Autodesk Inventor part; units mm, degrees
ref_plane "Work Plane1" through (0, 0, 0) normal (0, 0, 1) x (1, 0, 0)
ref_plane "YZ Plane" through (0, 0, 0) normal (1, 0, 0) x (0, 1, 0)
ref_plane "XZ Plane" through (0, 0, 0) normal (0, 1, 0) x (-1, 0, 0)
ref_plane "Work Plane1" through (0, 0, 0) normal (0, 0, 1) x (1, 0, 0)
sketch "Sketch1" plane through (0, 0, 0) normal (0, 0, 1) x (1, 0, 0)
  line L0 (27, 15) -> (27, 17)
  line L1 (21.5, 17) -> (26.5, 17) construction
  line L2 (22, 17) -> (22, 21.5)
  line L3 (27, 15) -> (27, 17)
  line L4 (21.5, 17) -> (26.5, 17)
  line L5 (21.5, 22) -> (7.7913, 22)
  line L6 (14, 22) -> (14, 26.5) construction
  line L7 (27, 15) -> (27, 17)
  line L8 (22, 17) -> (27, 17)
  line L9 (22, 17) -> (22, 21.5)
  line L10 (21.5, 22) -> (22, 22)
  line L11 (22, 22) -> (22, 21.5)
  line L12 (21.5, 22) -> (14, 22)
  line L13 (11.5, 27) -> (13.5, 27)
  line L14 (7.7913, 22) -> (21.5, 22)
  line L15 (27, 15) -> (27, 0)
  line L16 (14, 22) -> (14, 24)
  line L17 (14, 24) -> (27, 24)
  line L18 (27, 24) -> (29, 24)
  line L19 (29, -16) -> (29, 24)
  line L20 (29, -16) -> (-6, -16)
  line L21 (-6, -16) -> (-6, -14)
  line L22 (-6, -14) -> (27, -14)
  line L23 (27, -14) -> (27, 0)
  point P0 (0, 0)
  dimension "d0" = 2
  dimension "d1" = 2
  dimension "d2" = 40
  dimension "d3" = 35
  dimension "d4" = 2
extrude "Extrusion1" add sketch "Sketch1" along normal blind 10 and the other way blind 21
sketch "Sketch2" plane through (14, 24, 10) normal (0, 1, 0) x (1, 0, 0)
  arc A0 (-3.601, 18) -> (-3.601, 13) centre (-8.5, 15.5) ccw
  arc A1 (-3.601, 18) -> (-3.601, 13) centre (-8.5, 15.5) ccw
  arc A2 (-2.5, 13) -> (-2.5, 18) centre (-2.5, 15.5) ccw
  line L0 (-2.5, 13) -> (-3.601, 13)
  line L1 (-2.5, 18) -> (-3.601, 18)
  arc A3 (-2.5, 13) -> (-2.5, 18) centre (-2.5, 15.5) ccw
  line L2 (-3.601, 13) -> (-2.5, 13)
  line L3 (-3.601, 18) -> (-2.5, 18)
  line L4 (0.5, 15.5) -> (0.5, 0)
  line L5 (15, 0) -> (0, 0)
  line L6 (0.5, 15.5) -> (0.5, 31)
  line L7 (0, 31) -> (0, 0)
  line L8 (13, 0) -> (-20, 0)
  line L9 (0.5, 0) -> (-20, 0)
  line L10 (-20, 31) -> (-20, 0)
  line L11 (-20, 0) -> (-20, 31)
  line L12 (-20, 31) -> (0.5, 31)
  point P0 (-14, 10)
  point P1 (0, 15.5)
extrude "Extrusion2" add sketch "Sketch2" against normal blind 2 contours L7 L8 L10 L12
sketch "Sketch3" plane through (22, 17, 10) normal (0, -1, 0) x (1, 0, 0)
  arc A0 (3.799, -14.75) -> (3.799, -16.25) centre (2.5, -15.5) ccw
  circle A1 centre (2.5, -15.5) radius 1.5
  point P0 (-22, -10)
  point P1 (3.799, -16.25)
  point P2 (3.799, -14.75)
extrude "Extrusion3" cut sketch "Sketch3" against normal blind 17
sketch "Sketch4" plane through (29, -16, 10) normal (1, 0, 0) x (0, 0, -1)
  line L0 (13, 40) -> (18, 40)
  line L1 (15.5, 40) -> (15.5, 21)
  circle A0 centre (15.5, 21) radius 2.3
  point P0 (10, 16)
  dimension "d15" = 19
  dimension "d16" = 4.6
extrude "Extrusion4" cut sketch "Sketch4" against normal blind 2
sketch "Sketch5" plane through (29, -16, 10) normal (1, 0, 0) x (0, 0, -1)
  circle A0 centre (21.9497, 21.0658) radius 0.6
  circle A1 centre (9.0503, 20.9342) radius 0.6
  circle A2 centre (15.4342, 27.4497) radius 0.6
  circle A3 centre (15.5699, 14.1504) radius 0.6
  circle A4 centre (15.4342, 27.4497) radius 1
  circle A5 centre (21.9497, 21.0658) radius 1
  circle A6 centre (15.5699, 14.1504) radius 1
  circle A7 centre (9.0503, 20.9342) radius 1
  point P0 (10, 16)
  dimension "d19" = 2
  dimension "d20" = 2
  dimension "d21" = 2
  dimension "d22" = 2
extrude "Extrusion5" cut sketch "Sketch5" against normal blind 2.1 contours A0 | A1 | A3 | A5 | A6 | A7
fillet "Fillet1" radius 2 4 edges at (27, -14, -5.5) (22, 17, -5.5) (29, 24, -5.5) (29, -16, -5.5)
fillet "Fillet2" radius 2 2 edges at (-6, -16, -5.5) (-6, 24, -5.5)
sketch "Sketch6" plane through (27, -16, -21) normal (0, -1, 0) x (1, 0, 0)
  circle A0 centre (-21.5, 15.5) radius 1.5
  circle A1 centre (-21.5, 15.5) radius 1.5
  point P0 (-27, 21)
extrude "Extrusion6" cut sketch "Sketch6" against normal blind 3
Input: part model. Units: mm. Frame: model coordinates. A direction names the side the tool comes from. Coordinates: 2 decimals unless noted, no trailing zeros. Loops run counter-clockwise (first coordinate to the right, second up) from the corner with the lowest first, then second, coordinate; pieces in that order, holes last.
Q1. Set-up query: faces 1 (the face through (11, 22, -9)), 2 (the face through (0.004, 23.014, -5.706)), 3 (the face through (28.014, 6.057, -11.82)). Return all of +Z, -Z, +X, -X, +Y, -Y with unobstructed straight access to the full face (end or side cutting, diameter ignored); none if empty.
Q2. Draft query along Z for faces 4 (the face through (28, 6, -21)), 5 (the face through (22.57, 17.6, -5.28)), 6 (the face through (28.014, 2.755, -5.001)). Return one class per face: +Z half, -Z half, draft (parallel to the pull), parting line (faces both ways), or undercut.
Q3. Cut plane B-B (x = 19). Output: boundary loops of the cut face in (y, z), then the cut area to 3 significant figures.
Q4. Contact query for flat-ended pins moving along their axis: pin 1 (0.9 mm diameter, centred on y = 21, z = -8.5, fed in from -X); pin 2 (8.5 mm diameter, centred on y = 1, z = -6, fed in from -X). Output: stop coordinate, or through.
Q5. Material intervals for line 1 (Y direction, x = 15.5, z = -13); line 2 (Y direction, x = 28.15, z = -5.5); line 3 (Z direction, x = 5.5, y = 22.95), sorted ascending.
Q6. Cut plane D-D (x = 24.5). Output: boundary loops of the cut face in (y, z).
Q7. Cut plane A-A (x = 5.5). Output: boundary loops of the cut face in (y, z).
Working result:
1. face 1: +Z, -Z, -X
1. face 2: +Y
1. face 3: +X, -X
2. face 4: -Z half
2. face 5: draft
2. face 6: undercut
3. outline: (-16, -21) - (-14, -21) - (-14, 10) - (-16, 10) - close; (22, -21) - (24, -21) - (24, 10) - (22, 10) - close
3. area: 124 mm2
4. pin 1: stops at x = 22
4. pin 2: stops at x = 27
5. line 1: y = -16 to -14, 22 to 24
5. line 2: y = -15.64 to -2.85, -0.85 to 2.7, 7.3 to 23.64
5. line 3: z = -21 to -11, 0 to 10
6. outline: (-16, -21) - (-14, -21) - (-14, 10) - (-16, 10) - close; (17, -21) - (24, -21) - (24, -7) - (17, -7) - close; (17, -4) - (24, -4) - (24, 10) - (17, 10) - close
7. outline: (-16, -21) - (-14, -21) - (-14, -7) - (-16, -7) - close; (-16, -4) - (-14, -4) - (-14, 10) - (-16, 10) - close; (22, -21) - (24, -21) - (24, -11) - (22, -11) - close; (22, 0) - (24, 0) - (24, 10) - (22, 10) - close
